```python
from build123d import *

# Parameters (mm, degrees)
SKETCH1_W           = 29.6418
SKETCH1_H           = 7
BOSS_EXTRUDE1_DEPTH = 21.6154
SKETCH2_R           = 1.524
BOSS_EXTRUDE2_DEPTH = 3.175
SKETCH3_R           = 2.5
CUT_EXTRUDE1_DEPTH  = 3.81


with BuildPart() as part:
    # Sketch1 → Boss-Extrude1 (new body)
    with BuildSketch(Plane.XY):
        with Locations((14.8209, 3.5)):
            Rectangle(SKETCH1_W, SKETCH1_H)
    extrude(amount=BOSS_EXTRUDE1_DEPTH)

    # Sketch2 → Boss-Extrude2 (add)
    with BuildSketch(Plane(origin=(0, 0, 0), x_dir=(-1, 0, 0), z_dir=(0, 0, -1))):
        with BuildLine():
            Line((-33.1724, 6), (3.5306, 6))
            ThreePointArc((3.5306, 6), (6.0306, 3.5), (3.5306, 1))
            Line((3.5306, 1), (-33.1724, 1))
            ThreePointArc((-33.1724, 1), (-35.6724, 3.5), (-33.1724, 6))
        make_face()
        with Locations((-33.1724, 3.5)):
            Circle(SKETCH2_R, mode=Mode.SUBTRACT)
        with Locations((3.5306, 3.5)):
            Circle(SKETCH2_R, mode=Mode.SUBTRACT)
    extrude(amount=-BOSS_EXTRUDE2_DEPTH)

    # Sketch3 → Cut-Extrude1 (cut)
    with BuildSketch(Plane.XY.offset(21.6154)):
        with Locations((6.8209, 3.5)):
            Circle(SKETCH3_R)
        with Locations((22.8209, 3.5)):
            Circle(SKETCH3_R)
    extrude(amount=-CUT_EXTRUDE1_DEPTH, mode=Mode.SUBTRACT)


solid = part.part
```
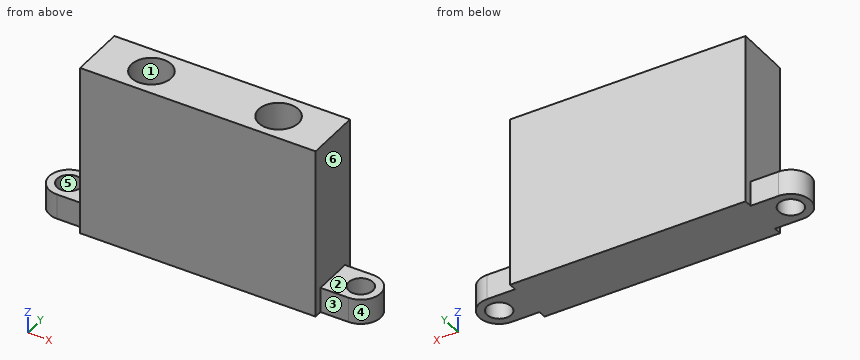
Build history of the part. All positions in model axes, mm. Face numbers are marked on the shaded views. A direction names the side the tool comes from. Coordinates: 2 decimals unless noted, no trailing zeros. Order: outer loops, then holes, each group sorted by start corner. A loop starts at its lowest first (then second) coordinate and runs counter-clockwise, first axis right, second up. Notation, with made-up numbers: (61.25, 53.5) -> (71.25, 53.5) arc R26 ccw to (71.25, 71.5) -> close; hole circle Ø9 at (55, 72.25). An arc over 180 degrees is marked (long way). Answer in a Markdown table with one row per item. Add a question column.
Q1. Mould opens along Y. For the marked faces 4, 5 and 6 say: +Y half, -Y half, draft (parallel to the pull), parting line (faces both ways), or undercut.
Q2. Band-saw the part on B-B, the plane z = 19.5. List the corners of the cut face in (x, y).
Q3. Band-saw the part on D-D, the plane y = 0.5. List the corners of the cut face in (x, z).
Q4. Which spindle directions (+Z, -Z, +X, -X, +Y, -Y) get a long thin tool onto all of the face, cutting with end or side? Do the marked faces 1, 2 and 3. Say none if no direction does.
Q5. Wall check: line 1 along X through (y, z) = (5.75, 13); line 2 along Z through (x, y) = (22.5, 3.75); line 3 along X through (y, z) = (4.5, 1.75). Give the ranges that are in metal, low to high. Write a range as [from, to].
Q6. Band-saw the part on A-A, the plane y = 3.5. List the corners of the cut face in (x, z) (3 decimals), then the cut area to 3 significant figures.
Q7. Drop flat-ended pins along their axis: pin 1 (2 mm diameter, centred on y = 1.5, z = 7.5, fed in from -X); pin 2 (1.5 mm diameter, centred on x = -1.5, z = 6, fed in from -Y); pin 3 (4 mm diameter, centred on x = 33.17, y = 3.5, fed in from +Z) (3 decimals); pin 4 (2 mm diameter, centred on y = 4, z = 11, fed in from +X). Give the stop position or say it passes through.
Q8. Band-saw the part on C-C, the plane x = 23. List the corners of the cut face in (y, z).
Answers follow:
| question | item | result |
|---|---|---|
| 1 | face 4 | parting line |
| 1 | face 5 | undercut |
| 1 | face 6 | draft |
| 2 | outline | (0, 0) -> (29.64, 0) -> (29.64, 7) -> (0, 7) -> close; hole circle Ø5 at (6.82, 3.5); hole circle Ø5 at (22.82, 3.5) |
| 3 | outline | (0, 0) -> (29.64, 0) -> (29.64, 21.62) -> (0, 21.62) -> close |
| 4 | face 1 | +Z |
| 4 | face 2 | +Z, +X, +Y, -Y |
| 4 | face 3 | +Z, -Z, +X, -Y |
| 5 | line 1 | [0, 29.64] |
| 5 | line 2 | [0, 17.81] |
| 5 | line 3 | [-5.82, -4.68], [-2.38, 32.02], [34.32, 35.46] |
| 6 | outline | (-6.031, 0) -> (-5.055, 0) -> (-5.055, 3.175) -> (-6.031, 3.175) -> close; (-2.007, 0) -> (31.648, 0) -> (31.648, 3.175) -> (29.642, 3.175) -> (29.642, 21.615) -> (25.321, 21.615) -> (25.321, 17.805) -> (20.321, 17.805) -> (20.321, 21.615) -> (9.321, 21.615) -> (9.321, 17.805) -> (4.321, 17.805) -> (4.321, 21.615) -> (0, 21.615) -> (0, 3.175) -> (-2.007, 3.175) -> close; (34.696, 0) -> (35.672, 0) -> (35.672, 3.175) -> (34.696, 3.175) -> close |
| 6 | area | 622 mm^2 |
| 7 | pin 1 | x = 0 |
| 7 | pin 2 | through |
| 7 | pin 3 | z = 3.175 |
| 7 | pin 4 | x = 29.64 |
| 8 | outline | (0, 0) -> (7, 0) -> (7, 21.62) -> (5.99, 21.62) -> (5.99, 17.81) -> (1.01, 17.81) -> (1.01, 21.62) -> (0, 21.62) -> close |
